Autodesk Inventor part; units mm, degrees
ref_plane "YZ Plane" through (0, 0, 0) normal (1, 0, 0) x (0, 1, 0)
ref_plane "XZ Plane" through (0, 0, 0) normal (0, 1, 0) x (-1, 0, 0)
sketch "Sketch1" plane through (0, 0, 0) normal (0, 0, 1) x (1, 0, 0)
  circle A0 centre (0, 0) radius 11.25
  line L0 (0, 0) -> (2.5, 0)
  circle A1 centre (2.5, 0) radius 7.5
  line L1 (8, 6.7455) -> (8, -7.7933)
  point P0 (10, 0)
  point P1 (10, 0)
  point P2 (8, -5.099)
  point P3 (8, 5.099)
  dimension "d2" = 15
  dimension "d0" = 22.5
  dimension "d1" = 2.5
  dimension "d3" = 2
extrude "Extrusion1" add sketch "Sketch1" along normal blind 2.5 contours A0 | A1 L1 | L1 A1
extrude "Extrusion2" add sketch "Sketch1" along normal blind 11 from surface at 2.5 contours L1 A1 picked at (-0.3888, 1.1518)
sketch "Sketch2" plane through (2.5, 0, 13.5) normal (0, 0, 1) x (1, 0, 0)
  line L0 (0, 0) -> (0, 3)
  circle A0 centre (0, 3) radius 2.75
  line L1 (-18.25, 0) -> (13.25, 0) construction
  circle A1 centre (0, -3) radius 2.75
  point P0 (-2.5, 0)
  dimension "d8" = 3
  dimension "d23" = 5.5
hole "Hole1" at (2.5, 3, 13.5) at (2.5, -3, 13.5) direction (0, 0, -1) diameter 3 depth 4
draft "FaceDraft1" angle 2.5 pull direction (0, 0, -1) faces at (11.1043, -1.8046, 1.6667) fixed edges at (-11.25, 0, 2.5)
sketch "Sketch3" plane through (0, 0, 20) normal (0, 0, 1) x (1, 0, 0)
  arc A0 (5.5, 4) -> (5.5, -4) centre (2.5, 0) ccw
  circle A1 centre (2.5, 2) radius 1.5
  circle A2 centre (2.5, -1.8526) radius 1.5
  line L0 (2.5, 5) -> (27.5, 5)
  line L1 (2.5, -5) -> (27.5, -5)
  line L2 (27.5, -5) -> (27.5, 5)
  point P0 (0, 0)
  dimension "d18" = 25
  dimension "d19" = 25
Could you check a few things on this model? Use its own coordinates, in mm. A direction names the side the tool comes from. Round coordinates to 2 decimals unless told otherwise and drop trailing zeros. Loops run counter-clockwise (first coordinate to the right, second up) from the corner with the lowest first, then second, coordinate; pieces in that order, holes last. Notation, with made-up numbers: (31, 64) - (55, 64) arc R36 cw to (55, 99) - close; hole circle Ø2 at (64.5, 5.25). An arc over 180 degrees is marked (long way). Write item = value, one per line.
1) If we mould it in two halves opening along X, with no side actions, what happens to faces 1 (the flat face through (-5.2, 0.2, 2.5)), 2 (the flat face through (8, 0, 8)), 3 (the flat face through (2, -3, 9.5)), 4 (the flat face through (2, 3, 9.5))? For each: pulls with the +X half, pulls with the -X half, needs draft (parallel to the pull), parting line crosses it, or undercut.
Computed:
face_1 = needs draft
face_2 = pulls with the +X half
face_3 = undercut
face_4 = undercut
2) On a 3-axis mill with a long thin cutter (end or side, diameter ignored), from which of +Z, -Z, +X, -X, +Y, -Y can I reach the whole of each face in a straight line? I mean faces 5 (the flat face through (1, 0, 13.5)), 6 (the cylindrical face through (-5, 0, 8)). Say none if no direction works.
Computed:
face_5 = +Z, +X, -X, +Y, -Y
face_6 = +Z
3) Imagine slicing it at C-C (x = 0). Please give me the cut outline in (y, z), and give its area (3 significant figures).
Computed:
outline = (-11.25, 2.5) - (-11.14, 0) - (11.14, 0) - (11.25, 2.5) - (7.07, 2.5) - (7.07, 13.5) - (-7.07, 13.5) - (-7.07, 2.5) - close
area = 212 mm2
4) I need wall thicknesses on line 1 along Y through (x, z) = (2.5, 11.1); line 2 along Z through (x, y) = (9.25, -3); line 3 along X through (y, z) = (3, 12.65). Which ranges of each line are inside material? Lowest first, please. Write a range as from..to.
Computed:
line_1 = -7.5..-4.5, -1.5..1.5, 4.5..7.5
line_2 = 0..2.5
line_3 = -4.37..1, 4..8
5) Imagine slicing it at D-D (z = 8.5). Please give me the cut outline in (x, y).
Computed:
outline = (8, -5.1) - (8, 5.1) arc R7.5 ccw (long way) to start
6) Imagine slicing it at B-B (z = 12.25). Please give me the cut outline in (x, y), and give its area (3 significant figures).
Computed:
outline = (8, -5.1) - (8, 5.1) arc R7.5 ccw (long way) to start; hole circle Ø3 at (2.5, -3); hole circle Ø3 at (2.5, 3)
area = 149 mm2
7) I'm going to push flat-ended pins straight in: P1, Ø4, axis at x = 2, z = 4, coming from the -Y side; P2, Ø4, axis at x = 3, z = 11, coming from the -Y side; P3, Ø2.5, axis at x = 2.5, y = -3, coming from the +Z side. Where does each tip first touch, or does it pass through?
Computed:
P1 = -11.23
P2 = -7.5
P3 = 9.5
8) Imagine slicing it at A-A (y = 0). Please give me the cut outline in (x, z), and give its area (3 significant figures).
Computed:
outline = (-11.25, 2.5) - (-11.14, 0) - (11.14, 0) - (11.25, 2.5) - (8, 2.5) - (8, 13.5) - (-5, 13.5) - (-5, 2.5) - close
area = 199 mm2
